from build123d import *

# Parameters (mm, degrees)
BOSS_EXTRUDE1_DEPTH   = 1.6
SKETCH2_R             = 3.45
BOSS_EXTRUDE2_DEPTH   = 1.4
M5X0_8_TAPPED_HOLE1_D = 4.2


with BuildPart() as part:
    # Sketch1 → Boss-Extrude1 (new body)
    with BuildSketch(Plane.XY):
        with BuildLine():
            Line((1.5, 0), (35.38, 0))
            ThreePointArc((35.38, 0), (36.440660172, 0.439339828), (36.88, 1.5))
            Line((36.88, 1.5), (36.88, 8.5))
            ThreePointArc((36.88, 8.5), (36.440660172, 9.560660172), (35.38, 10))
            Line((35.38, 10), (1.5, 10))
            ThreePointArc((1.5, 10), (0.439339828, 9.560660172), (0, 8.5))
            Line((0, 8.5), (0, 1.5))
            ThreePointArc((0, 1.5), (0.439339828, 0.439339828), (1.5, 0))
        make_face()
    extrude(amount=BOSS_EXTRUDE1_DEPTH)

    # Sketch2 → Boss-Extrude2 (add)
    with BuildSketch(Plane.XY.offset(1.6)):
        with Locations((8.44, 5)):
            Circle(SKETCH2_R)
        with Locations((28.44, 5)):
            Circle(SKETCH2_R)
    extrude(amount=BOSS_EXTRUDE2_DEPTH)

    # M5x0.8 Tapped Hole1 (through all)
    with Locations(Plane.XY.offset(3)):
        with Locations((8.44, 5), (28.44, 5)):
            Hole(M5X0_8_TAPPED_HOLE1_D / 2)


solid = part.part
Design review of the part built by this model. Coordinates are the model's own, in mm. A direction names the side the tool comes from. Give positions to 0.01 mm unless a question says otherwise; leave off trailing zeros. Order: outer loops, then holes, each group sorted by start corner. A loop starts at its lowest first (then second) coordinate and runs counter-clockwise, first axis right, second up. Notation, with made-up numbers: (37, 70.5) - (72, 70.5) arc R3 cw to (72, 74.5) - close; hole circle Ø1 at (89, -13.75). An arc over 180 degrees is marked (long way). Write item = value, one per line. Start each with the question number.
Q1. We need section D-D on z = 0.7. State the section outline as (x, y) points.
Q2. Tool access review of faces 1 (the face through (31.627, 3.679, 2.29)), 2 (the face through (18, 0, 1)): name each direction out of +Z, -Z, +X, -X, +Y, -Y from which nothing blocks a thin tool from reaching the whole face with its end or side.
Q3. We need section B-B on z = 2.5. State the section outline as (x, y) points, plus the area to 3 significant figures.
Q4. To check wall thickness, follow L1, parallel to Y at x = 28.44, z = 1.45; L2, parallel to X at y = 5.5, z = 1.9; L3, parallel to X at y = 6.5, z = 0.75. State the ranges of each line that lie inside material, in increasing order. Write a range as from..to.
Q5. We need section A-A on x = 8.44. State the section outline as (y, z) points.
Q6. Clearance check with a flat-ended pin moving along its axis: pin 1 Ø1.5 at (x, y) = (17, 6.5) entering from -Z. State where the tip first meets the part, or that it passes through.
Q7. Mouldability with a two-part tool opening along Y and no side actions: class faces 3 (the face through (9.988, 6.419, 1.479)), 4 (the face through (26.437, 5.631, 1.479)), 5 (the face through (31, 5, 3)), 6 (the face through (36.5, 9.5, 0.8)) as released by +Y, released by -Y, zero draft, split by the parting line, or undercut.
Q8. We need section C-C on y = 5. State the section outline as (x, z) points, plus the area to 3 significant figures.
Working result:
q1.outline = (0, 1.5) arc R1.5 ccw to (1.5, 0) - (35.38, 0) arc R1.5 ccw to (36.88, 1.5) - (36.88, 8.5) arc R1.5 ccw to (35.38, 10) - (1.5, 10) arc R1.5 ccw to (0, 8.5) - close; hole circle Ø4.2 at (8.44, 5); hole circle Ø4.2 at (28.44, 5)
q2.face_1 = +Z
q2.face_2 = +Z, -Z, +X, -X, -Y
q3.outline = circle Ø6.9 at (8.44, 5); circle Ø6.9 at (28.44, 5); hole circle Ø4.2 at (8.44, 5); hole circle Ø4.2 at (28.44, 5)
q3.area = 47.1 mm²
q4.L1 = 0..2.9, 7.1..10
q4.L2 = 5.03..6.4, 10.48..11.85, 25.03..26.4, 30.48..31.85
q4.L3 = 0..6.97, 9.91..26.97, 29.91..36.88
q5.outline = (0, 0) - (2.9, 0) - (2.9, 3) - (1.55, 3) - (1.55, 1.6) - (0, 1.6) - close; (7.1, 0) - (10, 0) - (10, 1.6) - (8.45, 1.6) - (8.45, 3) - (7.1, 3) - close
q6.pin_1 = 0
q7.face_3 = undercut
q7.face_4 = undercut
q7.face_5 = zero draft
q7.face_6 = released by +Y
q8.outline = (0, 0) - (6.34, 0) - (6.34, 3) - (4.99, 3) - (4.99, 1.6) - (0, 1.6) - close; (10.54, 0) - (26.34, 0) - (26.34, 3) - (24.99, 3) - (24.99, 1.6) - (11.89, 1.6) - (11.89, 3) - (10.54, 3) - close; (30.54, 0) - (36.88, 0) - (36.88, 1.6) - (31.89, 1.6) - (31.89, 3) - (30.54, 3) - close
q8.area = 53.1 mm²
